from build123d import *

# Parameters (mm, degrees)
SKETCH_W         = 59
SKETCH_H         = 52
PAD_DEPTH        = 9
SKETCH001_R      = 1.75
SKETCH001_R_2    = 2.5
PAD001_DEPTH     = 19
SKETCH002_W      = 52
SKETCH002_H      = 9
PAD002_DEPTH     = 6
HOLE_D           = 6.6
HOLE_DEPTH       = 25
HOLE_CSINK_D     = 12
HOLE_CSINK_ANGLE = 90
SKETCH004_W      = 59
SKETCH004_H      = 10
SKETCH004_H_2    = 12
POCKET_DEPTH     = 5
FILLET_R         = 3


with BuildPart() as part:
    # Sketch → Pad (new body)
    with BuildSketch(Plane.XY):
        with Locations((29.5, -26)):
            Rectangle(SKETCH_W, SKETCH_H)
    extrude(amount=PAD_DEPTH)

    # Sketch001 (on Face2 of Pad) → Pad001 (join)
    with BuildSketch(Plane.YZ.offset(59)):
        with Locations((-47, 4.5)):
            Circle(SKETCH001_R)
        with Locations((-5, 4.5)):
            Circle(SKETCH001_R)
        with Locations((-26, 4.5)):
            Circle(SKETCH001_R_2)
    extrude(amount=PAD001_DEPTH)

    # Sketch002 (on Face12 of Pad001) → Pad002 (join)
    with BuildSketch(Plane.YZ.offset(78)):
        with Locations((-26, 4.5)):
            Rectangle(SKETCH002_W, SKETCH002_H)
    extrude(amount=PAD002_DEPTH)

    # Hole
    with Locations(Plane.XY.offset(9)):
        with Locations((33, -16)):
            CounterSinkHole(HOLE_D / 2, HOLE_CSINK_D / 2, depth=HOLE_DEPTH, counter_sink_angle=HOLE_CSINK_ANGLE)

    # Sketch004 (on Face12 of Hole) → Pocket (cut)
    with BuildSketch(Plane(origin=(0, 0, 0), x_dir=(1, 0, 0), z_dir=(0, 0, -1))):
        with Locations((29.5, 16)):
            Rectangle(SKETCH004_W, SKETCH004_H)
        with Locations((29.5, 36.5)):
            Rectangle(SKETCH004_W, SKETCH004_H_2)
    extrude(amount=-POCKET_DEPTH, mode=Mode.SUBTRACT)

    # Fillet
    fillet_edges = [part.edges().sort_by_distance(p)[0] for p in [
        (29.5, 0, 0),
        (81, 0, 0),
        (29.5, -11, 0),
        (29.5, -21, 0),
        (29.5, -30.5, 0),
        (29.5, -42.5, 0),
        (29.5, -52, 0),
        (81, -52, 0),
    ]]
    fillet(fillet_edges, radius=FILLET_R)


solid = part.part
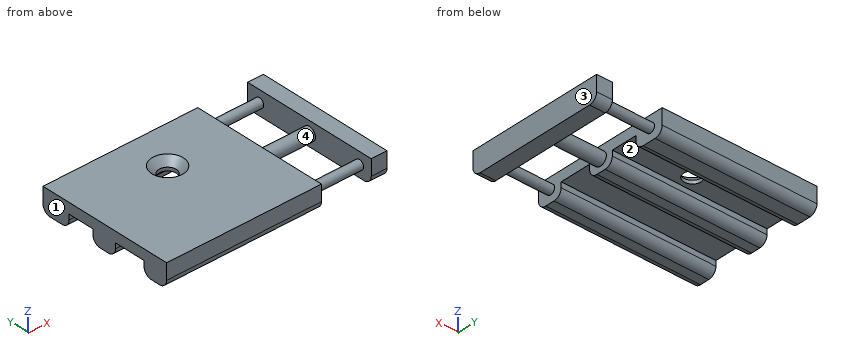
For this review, take the finished solid that the model builds, in its own axes (mm). Face numbers are marked on the shaded views. A direction names the side the tool comes from. Round coordinates to 2 decimals unless told otherwise and drop trailing zeros. Order: outer loops, then holes, each group sorted by start corner. A loop starts at its lowest first (then second) coordinate and runs counter-clockwise, first axis right, second up. Notation, with made-up numbers: (-36, 73.25) -> (-5, 73.25) arc R29 cw to (-5, 112.25) -> close; hole circle Ø3 at (38.25, 16). An arc over 180 degrees is marked (long way). Write item = value, one per line. Start each with the question number.
1) The part is to be moulded in two halves that separate along Y. For the marked faces 3 and 4, say which applies: +Y half, -Y half, draft (parallel to the pull), parting line (faces both ways), or undercut.
2) Take a section at B-B on x = 49. State the section outline as (y, z) points.
3) Take a section at A-A on y = -16. State the section outline as (x, z) points, plus the area to 3 significant figures.
4) Take a section at C-C on y = -47. State the section outline as (x, z) points, plus the area to 4 significant figures.
5) Take a section at D-D on x = 64.5. State the section outline as (y, z) points.
6) To check wall thickness, follow line 1 (Y direction, x = 45, z = 4); line 2 (X direction, y = -16, z = 5.65); line 3 (Y direction, x = 33, z = 5.6). State the ranges of each line that lie inside material, in increasing order. Write a range as from..to.
7) Tool access review of the marked faces 1 and 2: name each direction out of +Z, -Z, +X, -X, +Y, -Y from which nothing blocks a thin tool from reaching the whole face with its end or side.
8) Insertion check: pin 1 (5.5 mm diameter, centred on x = 33, y = -16, fed in from -Z); pin 2 (13 mm diameter, centred on x = 20, y = -36, fed in from -Z); pin 3 (3 mm diameter, centred on x = 66.5, z = 4.5, fed in from -Y); pin 4 (12 mm diameter, centred on x = 67, y = -32, fed in from -Z). Each pin has a flat end and moves straight along its axis. Give the tip position at first contact, or say it passes through.
Verdict:
q1.face_3 = draft
q1.face_4 = undercut
q2.outline = (-52, 3) arc R3 ccw to (-49, 0) -> (-45.5, 0) arc R3 ccw to (-42.5, 3) -> (-42.5, 5) -> (-30.5, 5) -> (-30.5, 3) arc R3 ccw to (-27.5, 0) -> (-24, 0) arc R3 ccw to (-21, 3) -> (-21, 5) -> (-11, 5) -> (-11, 3) arc R3 ccw to (-8, 0) -> (-3, 0) arc R3 ccw to (0, 3) -> (0, 9) -> (-52, 9) -> close
q3.outline = (0, 5) -> (29.7, 5) -> (29.7, 6.3) -> (27, 9) -> (0, 9) -> close; (36.3, 5) -> (59, 5) -> (59, 9) -> (39, 9) -> (36.3, 6.3) -> close; (78, 0) -> (84, 0) -> (84, 9) -> (78, 9) -> close
q3.area = 256 mm2
q4.outline = (0, 0) -> (59, 0) -> (59, 2.75) -> (78, 2.75) -> (78, 0) -> (84, 0) -> (84, 9) -> (78, 9) -> (78, 6.25) -> (59, 6.25) -> (59, 9) -> (0, 9) -> close
q4.area = 651.5 mm2
q5.outline = circle Ø3.5 at (-47, 4.5); circle Ø5 at (-26, 4.5); circle Ø3.5 at (-5, 4.5)
q6.line_1 = -52..-42.5, -30.5..-21, -11..0
q6.line_2 = 0..29.7, 36.3..59, 78..84
q6.line_3 = -52..-19.3, -12.7..0
q7.face_1 = +Z, -Z, -X, +Y, -Y
q7.face_2 = -Z, -X
q8.pin_1 = through
q8.pin_2 = 0.76
q8.pin_3 = -48.75
q8.pin_4 = 2
